Can you work these out from the model? Positions are in its coordinate system, mm. Face numbers are marked on the shaded views. A direction names the side the tool comes from. Coordinates: 2 decimals unless noted, no trailing zeros. Write each loop counter-clockwise with the first axis right and the second up, starting at its lowest first coordinate (ties: lowest second). Pieces come first, ordered by that corner, then holes.
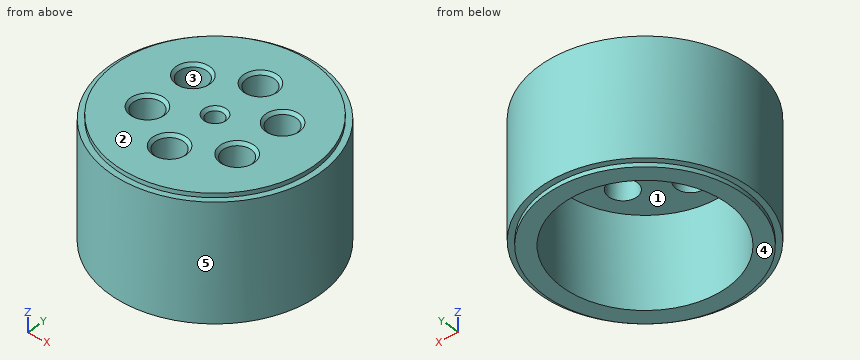
```python
from build123d import *

# Parameters (mm, degrees)
ESQUISSE1_R             = 34
ESQUISSE1_R_2           = 3
ESQUISSE1_R_3           = 5
BOSS_EXTRU_1_DEPTH      = 22
ESQUISSE2_R             = 37
ESQUISSE2_R_2           = 34
BOSS_EXTRU_2_DEPTH      = 44
ESQUISSE2_3_R           = 37
ESQUISSE2_3_R_2         = 34
ENL_V_MAT_EXTRU_1_DEPTH = 1.5
ESQUISSE3_R             = 35
ESQUISSE3_R_2           = 34
BOSS_EXTRU_3_DEPTH      = 1.5
CHANFREIN1_SIZE         = 1
ESQUISSE4_R             = 29
ENL_V_MAT_EXTRU_2_DEPTH = 32


with BuildPart() as part:
    # Esquisse1 → Boss.-Extru.1 (new body, symmetric)
    with BuildSketch(Plane.XY):
        Circle(ESQUISSE1_R)
        Circle(ESQUISSE1_R_2, mode=Mode.SUBTRACT)
        with Locations((0, 18.5)):
            Circle(ESQUISSE1_R_3, mode=Mode.SUBTRACT)
        with Locations((16.02146997, 9.25)):
            Circle(ESQUISSE1_R_3, mode=Mode.SUBTRACT)
        with Locations((16.02146997, -9.25)):
            Circle(ESQUISSE1_R_3, mode=Mode.SUBTRACT)
        with Locations((0, -18.5)):
            Circle(ESQUISSE1_R_3, mode=Mode.SUBTRACT)
        with Locations((-16.02146997, -9.25)):
            Circle(ESQUISSE1_R_3, mode=Mode.SUBTRACT)
        with Locations((-16.02146997, 9.25)):
            Circle(ESQUISSE1_R_3, mode=Mode.SUBTRACT)
    extrude(amount=BOSS_EXTRU_1_DEPTH, both=True)

    # Esquisse2 → Boss.-Extru.2 (add)
    with BuildSketch(Plane.XY.offset(22)):
        Circle(ESQUISSE2_R)
        Circle(ESQUISSE2_R_2, mode=Mode.SUBTRACT)
    extrude(amount=-BOSS_EXTRU_2_DEPTH)

    # Esquisse2_3 → Enl_v. mat.-Extru.1 (cut)
    with BuildSketch(Plane.XY.offset(22)):
        Circle(ESQUISSE2_3_R)
        Circle(ESQUISSE2_3_R_2, mode=Mode.SUBTRACT)
    enl_v_mat_extru_1 = extrude(amount=-ENL_V_MAT_EXTRU_1_DEPTH, mode=Mode.SUBTRACT)

    # Sym_trie1: Enl_v. mat.-Extru.1 across plane
    add(enl_v_mat_extru_1.mirror(Plane.XY), mode=Mode.SUBTRACT)

    # Esquisse3 → Boss.-Extru.3 (add)
    with BuildSketch(Plane.XY.offset(22)):
        Circle(ESQUISSE3_R)
        Circle(ESQUISSE3_R_2, mode=Mode.SUBTRACT)
    boss_extru_3 = extrude(amount=-BOSS_EXTRU_3_DEPTH)

    # Sym_trie2: Boss.-Extru.3 across plane
    add(boss_extru_3.mirror(Plane.XY))

    # Chanfrein1
    chanfrein1_edges = [part.edges().sort_by_distance(p)[0] for p in [
        (11.02146997, 9.25, -22),
        (11.02146997, 9.25, 22),
        (11.02146997, -9.25, -22),
        (11.02146997, -9.25, 22),
        (-5, -18.5, -22),
        (-5, -18.5, 22),
        (-21.02146997, -9.25, -22),
        (-21.02146997, -9.25, 22),
        (-21.02146997, 9.25, -22),
        (-21.02146997, 9.25, 22),
        (-3, 0, -22),
        (-3, 0, 22),
        (-5, 18.5, -22),
        (-5, 18.5, 22),
    ]]
    chamfer(chanfrein1_edges, length=CHANFREIN1_SIZE)

    # Esquisse4 → Enl_v. mat.-Extru.2 (cut)
    with BuildSketch(Plane(origin=(0, 0, -22), x_dir=(-1, 0, 0), z_dir=(0, 0, -1))):
        Circle(ESQUISSE4_R)
    extrude(amount=-ENL_V_MAT_EXTRU_2_DEPTH, mode=Mode.SUBTRACT)


solid = part.part
```
1. If we section it at D-D, the plane z = -1: List the corners of the cut face in (x, y) for me.
2. If we section it at A-A, the plane z = 16.5: List the corners of the cut face in (x, y) for me.
3. Which directions (+Z, -Z, +X, -X, +Y, -Y) give clear straight access to the entire face, cutting with the end or side of a thin tool? Please do the marked faces 1 and 2.
4. I'm going to push flat-ended pins straight in: P1, Ø4, axis at y = 3.5, z = -4, coming from the +X side; P2, Ø16, axis at x = -16.02, y = 9.25, coming from the -Z side; P3, Ø5, axis at x = -6.5, z = -6.5, coming from the -Y side; P4, Ø8, axis at y = 2.5, z = 2.5, coming from the -X side. Where does each tip first touch, or does it pass through?
5. If we section it at B-B, the plane y = -18.5: List the corners of the cut face in (x, z) for me.
6. If I drill on L1, parallel to Y at x = 0, z = 18; L2, parallel to Y at x = 0, z = -7; L3, parallel to Y at x = 13, z = 19, over which ranges is the centre line in solid material (lowest first)?
7. If we section it at C-C, the plane y = 9.25: List the corners of the cut face in (x, z) for me, plus the area to 3 significant figures.
8. We'd pull the mould along X, two halves only. Please class the marked faces 3, 4 and 5: released by +X, released by -X, zero draft, split by the parting line, or undercut.
Answers:
1. outline: circle Ø74 at (0, 0); hole circle Ø58 at (0, 0)
2. outline: circle Ø74 at (0, 0); hole circle Ø10 at (-16.02, -9.25); hole circle Ø10 at (-16.02, 9.25); hole circle Ø10 at (0, -18.5); hole circle Ø10 at (0, 18.5); hole circle Ø6 at (0, 0); hole circle Ø10 at (16.02, -9.25); hole circle Ø10 at (16.02, 9.25)
3. face 1: -Z
3. face 2: +Z, +X, -X, +Y, -Y
4. P1: stops at x = 36.97
4. P2: stops at z = 10
4. P3: stops at y = -36.78
4. P4: stops at x = -37
5. outline: (-32.04, -20.5) - (-29.71, -20.5) - (-29.71, -22) - (-22.33, -22) - (-22.33, 10) - (-5, 10) - (-5, 21) - (-6, 22) - (-29.71, 22) - (-29.71, 20.5) - (-32.04, 20.5) - close; (5, 10) - (22.33, 10) - (22.33, -22) - (29.71, -22) - (29.71, -20.5) - (32.04, -20.5) - (32.04, 20.5) - (29.71, 20.5) - (29.71, 22) - (6, 22) - (5, 21) - close
6. L1: y = -37 to -23.5, -13.5 to -3, 3 to 13.5, 23.5 to 37
6. L2: y = -37 to -29, 29 to 37
6. L3: y = -34.64 to -13.23, -5.27 to 5.27, 13.23 to 34.64
7. outline: (-35.83, -20.5) - (-33.76, -20.5) - (-33.76, -22) - (-27.49, -22) - (-27.49, 10) - (-21.02, 10) - (-21.02, 21) - (-22.02, 22) - (-33.76, 22) - (-33.76, 20.5) - (-35.83, 20.5) - close; (-11.02, 10) - (11.02, 10) - (11.02, 21) - (10.02, 22) - (-10.02, 22) - (-11.02, 21) - close; (21.02, 10) - (27.49, 10) - (27.49, -22) - (33.76, -22) - (33.76, -20.5) - (35.83, -20.5) - (35.83, 20.5) - (33.76, 20.5) - (33.76, 22) - (22.02, 22) - (21.02, 21) - close
7. area: 1,140 mm2
8. face 3: undercut
8. face 4: zero draft
8. face 5: split by the parting line
